Autodesk Inventor part; units mm, degrees
ref_plane "YZ Plane" through (0, 0, 0) normal (1, 0, 0) x (0, 1, 0)
ref_plane "XZ Plane" through (0, 0, 0) normal (0, 1, 0) x (-1, 0, 0)
ref_plane "XY Plane" through (0, 0, 0) normal (0, 0, 1) x (1, 0, 0)
sketch "Sketch1" plane through (0, 0, 0) normal (0, 1, 0) x (-1, 0, 0)
  arc A0 (29.684, 4.343) -> (29.5804, -5) centre (0, 0) ccw
  line L0 (29.5804, -5) -> (0, -5)
  line L1 (0, -5) -> (0, 4.343)
  line L2 (0, 4.343) -> (29.684, 4.343)
  dimension "d0" = 60
extrude "Extrusion1" add sketch "Sketch1" along normal blind 15
fillet "Fillet1" radius 2 2 edges at (29.9982, 15, 0.3325) (29.9982, 0, 0.3325)
properties part number "Hammer" material "Iron, Malleable"
Check sheet for the modelled part. Datum: model origin and axes. Units: mm. A direction names the side the tool comes from. Round coordinates to 2 decimals unless told otherwise and drop trailing zeros. Loops run counter-clockwise (first coordinate to the right, second up) from the corner with the lowest first, then second, coordinate; pieces in that order, holes last. Notation, with made-up numbers: (46.5, 34.25) - (86.5, 34.25) arc R15 ccw to (86.5, 47.25) - close; hole circle Ø11 at (-15, 45). An arc over 180 degrees is marked (long way). Answer as a JSON object with one key per item and string values. Group by question number.
Q1. Sectioned sample at A-A, the plane y = 12.25. Enter the section's corners in (x, z).
Q2. Scan lines: line 1 along Z through (x, y) = (-25.5, 13.5); line 2 along Z through (x, y) = (-25, 11.25); line 3 along Z through (x, y) = (25, 2.75). Record each from-to range of solid material in increasing order. Write a range as [from, to].
Q3. Mould release check, pull along Z, two halves, no side actions. Record for faces 1 (the face through (1, 15, 0)), 2 (the face through (-15, 7, -5)), 3 (the face through (29.986, 7.423, -0.921)): released by +Z, released by -Z, zero draft, split by the parting line, or undercut.
Q4. Set-up check for faces 4 (the face through (1, 0, 0)), 5 (the face through (0, 7, 0)): record each of +Z, -Z, +X, -X, +Y, -Y from which the full face is reachable in a straight line by a thin tool's end or side.
Q5. Gauge pin test, flat ends, axial feed: P1, Ø4.5, axis at x = -13.5, y = 7.5, coming from the +Z side; P2, Ø1.5, axis at x = -4.5, y = 11, coming from the -Z side; P3, Ø1.5, axis at x = -8, y = 10.5, coming from the -Z side. Record the tip position at first contact, or that the pin passes through.
Solution:
{
 "1": {"outline": "(-29.68, 4.34) - (0, 4.34) - (0, -5) - (-29.58, -5) arc R30 ccw (long way) to start"},
 "2": {"line 1": "z = [-15.68, -5], [4.34, 15.68]", "line 2": "z = [-16.58, -5], [4.34, 16.58]", "line 3": "z = [-16.58, 16.58]"},
 "3": {"face 1": "zero draft", "face 2": "undercut", "face 3": "split by the parting line"},
 "4": {"face 4": "+Z, -Z, +X, -X, -Y", "face 5": "-X, +Y, -Y"},
 "5": {"P1": "stops at z = 27.81", "P2": "stops at z = -29.76", "P3": "stops at z = -29.11"}
}
